Input: dimensioned drawing with shaded views. Units: mm. Origin: part minimum x, y, z. A direction names the side the tool comes from. Round coordinates to 2 decimals unless told otherwise and drop trailing zeros. Write each loop counter-clockwise with the first axis right and the second up, starting at its lowest first coordinate (ties: lowest second). Pieces come first, ordered by that corner, then holes. Notation, with made-up numbers: M -23.5,38.5 L 26.5,38.5 A22 ccw 26.5,72.5 Z; hole C 1,74.5 d5. An arc over 180 degrees is marked long. Answer in a Markdown table with one row per item. Add a question column.
Item 1: Cut plane C-C on z = 35.5. Return loops of the section in (x, y).
Item 2: Material intervals for probe 1 along Z at (x, y) = (40, 8.75); probe 2 along Z at (x, y) = (50, 2.75); probe 3 along Y at (x, z) = (40, 34), sorted ascending.
Item 3: Cut plane B-B on y = 3.5. Return loops of the section in (x, z) (1 decimal), and give its area (3 significant figures).
Item 4: Contact query for flat-ended pins moving along their axis: pin 1 (5 mm diameter, centred on x = 40, y = 10.5, fed in from +Z); pin 2 (5 mm diameter, centred on x = 68.5, y = 2, fed in from -Z); pin 3 (1.9 mm diameter, centred on x = 39.5, y = 4, fed in from +Z). Output: stop coordinate, or through.
Item 5: Cut plane D-D on x = 70. Return loops of the section in (y, z), and give its area (3 significant figures).
Item 6: Set-up query: the marked faces 1 and 2. Return all of +Z, -Z, +X, -X, +Y, -Y with unobstructed straight access to the full face (end or side cutting, diameter ignored); none if empty.
Item 7: Cut plane A-A on x = 40. Return loops of the section in (y, z), and give its area (3 significant figures).
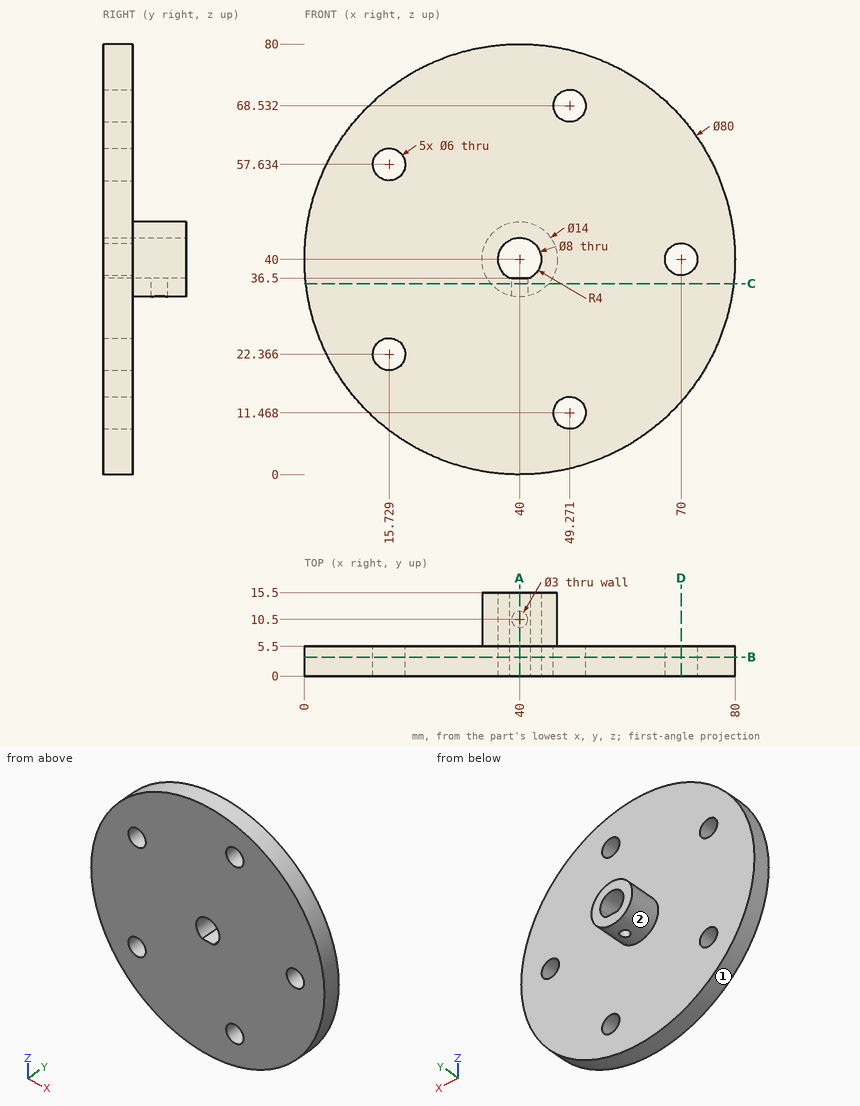
Results below:
| question | item | result |
|---|---|---|
| 1 | outline | M 0.25,0 L 79.75,0 L 79.75,5.5 L 45.36,5.5 L 45.36,15.5 L 34.64,15.5 L 34.64,5.5 L 0.25,5.5 Z; hole C 40,10.5 d3 |
| 2 | probe 1 | 33 to 36.5, 44 to 47 |
| 2 | probe 2 | 1.27 to 8.56, 14.38 to 65.62, 71.44 to 78.73 |
| 2 | probe 3 | 0 to 9, 12 to 15.5 |
| 3 | outline | C 40,40 d80; hole C 15.7,22.4 d6; hole C 15.7,57.6 d6; hole M 38.1,36.5 L 41.9,36.5 A4 ccw long Z; hole C 49.3,11.5 d6; hole C 49.3,68.5 d6; hole C 70,40 d6 |
| 3 | area | 4,840 mm2 |
| 4 | pin 1 | z = 47 |
| 4 | pin 2 | z = 9.6 |
| 4 | pin 3 | z = 80 |
| 5 | outline | M 0,13.54 L 5.5,13.54 L 5.5,37 L 0,37 Z; M 0,43 L 5.5,43 L 5.5,66.46 L 0,66.46 Z |
| 5 | area | 258 mm2 |
| 6 | face 1 | +Y, -Y |
| 6 | face 2 | +Y |
| 7 | outline | M 0,0 L 5.5,0 L 5.5,33 L 9,33 L 9,36.5 L 0,36.5 Z; M 0,44 L 15.5,44 L 15.5,47 L 5.5,47 L 5.5,80 L 0,80 Z; M 12,33 L 15.5,33 L 15.5,36.5 L 12,36.5 Z |
| 7 | area | 453 mm2 |
